Geometry check sheet. Reference: the model listing, model coordinates, mm. Round coordinates to 2 decimals unless told otherwise and drop trailing zeros. Write each loop counter-clockwise with the first axis right and the second up, starting at its lowest first coordinate (ties: lowest second). Pieces come first, ordered by that corner, then holes. Notation, with made-up numbers: (40.25, 2) -> (74.25, 2) arc R16 ccw to (74.25, 27) -> close; hole circle Ø2 at (44, 80). An arc over 180 degrees is marked (long way). Use a Markdown table: item, result.
```python
from build123d import *

# Parameters (mm, degrees)
F0_W     = 88.9
F0_H     = 38.1
F1_DEPTH = 203.2
F2_R     = 6.35
F3_SIZE  = 6.35
F4_SIZE  = 6.35
F6_DEPTH = 38.1
F7_R     = 6.35
F8_DEPTH = 2.54


with BuildPart() as f1:
    # F0 (on Front) → F1 (new body)
    with BuildSketch(Plane.XZ):
        Rectangle(F0_W, F0_H)
    extrude(amount=F1_DEPTH)

    # F2
    f2_edges = [f1.edges().sort_by_distance(p)[0] for p in [
        (-44.45, -101.6, 19.05),
        (-44.45, -101.6, -19.05),
        (44.45, -101.6, 19.05),
        (44.45, -101.6, -19.05),
    ]]
    fillet(f2_edges, radius=F2_R)

    # F3
    f3_edges = [f1.edges().sort_by_distance(p)[0] for p in [
        (0, -203.2, 19.05),
    ]]
    chamfer(f3_edges, length=F3_SIZE)

    # F4
    f4_edges = [f1.edges().sort_by_distance(p)[0] for p in [
        (0, 0, 19.05),
    ]]
    chamfer(f4_edges, length=F4_SIZE)

    # F5 (on face) → F6 (cut)
    with BuildSketch(Plane.YZ.offset(44.45)):
        Polygon((-46.870606, -50.8), (-76.2, 0), (-156.845, 0), (-186.174394, -50.8), align=None)
        Polygon((-156.845, 0), (-76.2, 0), (-46.870606, 50.8), (-186.174394, 50.8), align=None)
    extrude(amount=-F6_DEPTH, mode=Mode.SUBTRACT)

    # F7 (on face) → F8 (cut)
    with BuildSketch(Plane(origin=(0, 0, 0), x_dir=(-1, 0, 0), z_dir=(0, 1, 0))):
        with Locations((25.4, 0)):
            Circle(F7_R)
    extrude(amount=-F8_DEPTH, mode=Mode.SUBTRACT)


solid = f1.part
```
(1) Section check A-A on y = -91. Record the cut outline in (x, z).
A:
| item | result |
|---|---|
| outline | (-44.45, -12.7) arc R6.35 ccw to (-38.1, -19.05) -> (6.35, -19.05) -> (6.35, 19.05) -> (-38.1, 19.05) arc R6.35 ccw to (-44.45, 12.7) -> close |
(2) Gauge pin test, flat end, axial feed: pin 1 Ø6 at (y, z) = (-87.5, 0) entering from +X. Record the tip position at first contact, or that the pin passes through.
A:
| item | result |
|---|---|
| pin 1 | stops at x = 6.35 |
(3) Section check B-B on z = 3. Record the cut outline in (x, y).
A:
| item | result |
|---|---|
| outline | (-44.45, -196.85) -> (-38.1, -203.2) -> (38.1, -203.2) -> (44.45, -196.85) -> (44.45, -158.58) -> (6.35, -158.58) -> (6.35, -74.47) -> (44.45, -74.47) -> (44.45, -6.35) -> (38.1, 0) -> (-19.8, 0) -> (-19.8, -2.54) -> (-31, -2.54) -> (-31, 0) -> (-38.1, 0) -> (-44.45, -6.35) -> close |
(4) Thickness scan on line 1 (X direction, y = -101.5, z = -5); line 2 (Y direction, x = 12, z = -4.5). Record the ranges inside material, lowest first.
A:
| item | result |
|---|---|
| line 1 | x = -44.45 to 6.35 |
| line 2 | y = -203.2 to -159.44, -73.6 to 0 |
(5) Release check for a two-part mould opening along Z. For faces 1 (the face through (-40.35, -3.22, -15)), 2 (the face through (-40.4, -3.22, 14.95)), 3 (the face through (-19.056, -1.252, 0.279)) record: +Z half, -Z half, draft (parallel to the pull), parting line (faces both ways), or undercut.
A:
| item | result |
|---|---|
| face 1 | -Z half |
| face 2 | +Z half |
| face 3 | undercut |
